Design review of the part built by this model. Coordinates are the model's own, in mm. A direction names the side the tool comes from. Coordinates: 2 decimals unless noted, no trailing zeros. Write each loop counter-clockwise with the first axis right and the second up, starting at its lowest first coordinate (ties: lowest second). Pieces come first, ordered by that corner, then holes. Notation, with made-up numbers: M 83.25,76 L 127.25,76 A29 ccw 127.25,105 Z; hole C 83.25,26 d10. An arc over 180 degrees is marked long. Write item = value, one per line.
```python
from build123d import *


with BuildPart() as part:
    # Sketch1 → Revolve1 (revolve)
    with BuildSketch(Plane(origin=(0, 0, 0), x_dir=(0, 0, -1), z_dir=(1, 0, 0))):
        with BuildLine():
            Line((-10, 0), (-3, 0))
            Line((-3, 0), (13, 0))
            Line((13, 0), (13, 5.6))
            Line((13, 5.6), (5, 5.6))
            Line((5, 5.6), (3, 5.460146376))
            Line((3, 5.460146376), (3, 5))
            Line((3, 5), (-3, 5))
            Line((-3, 5), (-3, 3.5))
            Line((-3, 3.5), (-5, 3.5))
            Line((-5, 3.5), (-5, 5))
            Line((-5, 5), (-8, 5))
            Line((-8, 5), (-9.5, 4.868767005))
            ThreePointArc((-9.5, 4.868767005), (-9.853553391, 4.722320395), (-10, 4.368767005))
            Line((-10, 4.368767005), (-10, 0))
        make_face()
    revolve1 = revolve(axis=Axis((0, 0, 3), (0, 0, -1)))

    # Mirror1: Revolve1 across plane
    add(revolve1.mirror(Plane(origin=(0, 0, -13), x_dir=(1, 0, 0), z_dir=(0, 0, -1))))


solid = part.part
```
Q1. Machinability: for faces 4 (the cylindrical face through (-4.88, -1.08, -26.04)), 5 (the cylindrical face through (-4.88, -1.08, 0.04)), 6 (the flat face through (-3.3, -2.2, -31)), 7 (the flat face through (0, 0, -36)), which of the approach directions +Z, -Z, +X, -X, +Y, -Y give a long, thin tool a straight path to every point of the face, cutting with its end or side? Answer none if there is none.
Check result:
face_4 = -Z
face_5 = +Z
face_6 = none
face_7 = -Z, +X, -X, +Y, -Y
Q2. Wall thickness on line 1 (Z direction, x = -3, y = -2); line 2 (Z direction, x = -2.5, y = -4.5); line 3 (Z direction, x = 4.25, y = 2.25): over which ranges is each line inside the solid? List them lowest first.
Check result:
line_1 = -36 to -31, -29 to 3, 5 to 10
line_2 = -23 to -3
line_3 = -35.74 to -31, -29 to 3, 5 to 9.74
Q3. The part is to be moulded in two halves that separate along Z. For faces 1 (the flat face through (-3.3, -2.2, 5)), 2 (the cylindrical face through (-4.88, -1.08, -32.52)), 3 (the conical face through (-5.367, -1.192, -22.458)), say which applies: +Z half, -Z half, draft (parallel to the pull), parting line (faces both ways), or undercut.
Check result:
face_1 = undercut
face_2 = draft
face_3 = -Z half
Q4. Consider section B-B, the plane z = 3.5. State the section outline as (x, y) points, and give its area (3 significant figures).
Check result:
outline = C 0,0 d7
area = 38.5 mm²
Q5. For P1, Ø6, axis at x = -4, z = -19.5, coming from the +Y side; P2, Ø6, axis at x = 4, z = -25, coming from the +Y side, all flat-tipped, find the tip position at first contact; note any pin that passes through.
Check result:
P1 = 5.51
P2 = 5.17
Q6. Consider section A-A, the plane z = -1.5. State the section outline as (x, y) points, and give its area (3 significant figures).
Check result:
outline = C 0,0 d10
area = 78.5 mm²
